Input: part model. Units: mm. Frame: model coordinates. A direction names the side the tool comes from. Round coordinates to 2 decimals unless told otherwise and drop trailing zeros. Order: outer loops, then holes, each group sorted by start corner. A loop starts at its lowest first (then second) coordinate and runs counter-clockwise, first axis right, second up. Notation, with made-up numbers: (35.5, 5.25) -> (86.5, 5.25) arc R8 ccw to (86.5, 14.25) -> close; hole circle Ø2 at (53, 28). An arc over 180 degrees is marked (long way). Use a Markdown table: item, result.
from build123d import *

# Parameters (mm, degrees)
F2_DEPTH = 2.032
F3_DEPTH = 2.54
F5_DEPTH = 25.4
F7_DEPTH = 25.4


with BuildPart() as f2:
    # F0 (on Front) → F2 (new body)
    with BuildSketch(Plane.XZ):
        with BuildLine():
            ThreePointArc((246.888, 191.262), (241.308384, 204.732384), (227.838, 210.312))
            Line((227.838, 210.312), (-227.838, 210.312))
            ThreePointArc((-227.838, 210.312), (-241.308384, 204.732384), (-246.888, 191.262))
            Line((-246.888, 191.262), (-246.888, -191.262))
            ThreePointArc((-246.888, -191.262), (-241.308384, -204.732384), (-227.838, -210.312))
            Line((-227.838, -210.312), (227.838, -210.312))
            ThreePointArc((227.838, -210.312), (241.308384, -204.732384), (246.888, -191.262))
            Line((246.888, -191.262), (246.888, 191.262))
        make_face()
    extrude(amount=F2_DEPTH)

    # F1 (on Front) → F3 (cut)
    with BuildSketch(Plane.XZ):
        with BuildLine():
            Line((223.774, 206.248), (-223.774, 206.248))
            ThreePointArc((-223.774, 206.248), (-237.244384, 200.668384), (-242.824, 187.198))
            Line((-242.824, 187.198), (-242.824, -105.918))
            ThreePointArc((-242.824, -105.918), (-237.244384, -119.388384), (-223.774, -124.968))
            Line((-223.774, -124.968), (223.774, -124.968))
            ThreePointArc((223.774, -124.968), (237.244384, -119.388384), (242.824, -105.918))
            Line((242.824, -105.918), (242.824, 187.198))
            ThreePointArc((242.824, 187.198), (237.244384, 200.668384), (223.774, 206.248))
        make_face()
    extrude(amount=F3_DEPTH, mode=Mode.SUBTRACT)

    # F4 (on Front) → F5 (cut)
    with BuildSketch(Plane.XZ):
        Polygon((-230.124, -134.664931), (-236.474, -134.664931), (-160.274, -200.704931), (-153.924, -200.704931), align=None)
        Polygon((-211.074, -134.664931), (-217.424, -134.664931), (-160.274, -184.194931), (-153.924, -184.194931), align=None)
        Polygon((-230.124, -152.281931), (-236.474, -152.281931), (-180.601308, -200.704931), (-174.251308, -200.704931), align=None)
        Polygon((-230.124, -168.226628), (-236.474, -168.226628), (-198.999035, -200.704931), (-192.649035, -200.704931), align=None)
        Polygon((-230.124, -183.399803), (-236.474, -183.399803), (-216.506545, -200.704931), (-210.156545, -200.704931), align=None)
        Polygon((-160.274, -169.990187), (-153.924, -169.990187), (-194.683911, -134.664931), (-201.033911, -134.664931), align=None)
        Polygon((-160.274, -155.138477), (-153.924, -155.138477), (-177.547322, -134.664931), (-183.897322, -134.664931), align=None)
        Polygon((160.274, -184.194931), (217.424, -134.664931), (211.074, -134.664931), (153.924, -184.194931), align=None)
        Polygon((160.274, -200.704931), (236.474, -134.664931), (230.124, -134.664931), (153.924, -200.704931), align=None)
        Polygon((160.274, -169.990187), (201.033911, -134.664931), (194.683911, -134.664931), (153.924, -169.990187), align=None)
        Polygon((177.547322, -134.664931), (153.924, -155.138477), (160.274, -155.138477), (183.897322, -134.664931), align=None)
        Polygon((198.999035, -200.704931), (236.474, -168.226628), (230.124, -168.226628), (192.649035, -200.704931), align=None)
        Polygon((230.124, -152.281931), (174.251308, -200.704931), (180.601308, -200.704931), (236.474, -152.281931), align=None)
        Polygon((230.124, -183.399803), (210.156545, -200.704931), (216.506545, -200.704931), (236.474, -183.399803), align=None)
    extrude(amount=F5_DEPTH, mode=Mode.SUBTRACT)

    # F6 (on Front) → F7 (cut)
    with BuildSketch(Plane.XZ):
        with BuildLine():
            ThreePointArc((278.867032, 134.112), (282.463983, 140.014539), (283.718, 146.812))
            ThreePointArc((283.718, 146.812), (257.870539, 164.607983), (250.468968, 134.112))
            ThreePointArc((250.468968, 134.112), (264.668, 140.462), (278.867032, 134.112))
        make_face()
        with BuildLine():
            ThreePointArc((278.867032, 134.112), (264.668, 127.762), (250.468968, 134.112))
            ThreePointArc((250.468968, 134.112), (245.618, 121.412), (250.468968, 108.712))
            ThreePointArc((250.468968, 108.712), (264.668, 115.062), (278.867032, 108.712))
            ThreePointArc((278.867032, 108.712), (282.463983, 114.614539), (283.718, 121.412))
            ThreePointArc((283.718, 121.412), (282.463983, 128.209461), (278.867032, 134.112))
        make_face()
        with BuildLine():
            ThreePointArc((278.867032, 108.712), (264.668, 102.362), (250.468968, 108.712))
            ThreePointArc((250.468968, 108.712), (257.870539, 78.216017), (283.718, 96.012))
            ThreePointArc((283.718, 96.012), (282.463983, 102.809461), (278.867032, 108.712))
        make_face()
        with BuildLine():
            ThreePointArc((-250.468968, 134.112), (-246.872017, 140.014539), (-245.618, 146.812))
            ThreePointArc((-245.618, 146.812), (-271.465461, 164.607983), (-278.867032, 134.112))
            ThreePointArc((-278.867032, 134.112), (-264.668, 140.462), (-250.468968, 134.112))
        make_face()
        with BuildLine():
            ThreePointArc((-250.468968, 134.112), (-264.668, 127.762), (-278.867032, 134.112))
            ThreePointArc((-278.867032, 134.112), (-283.718, 121.412), (-278.867032, 108.712))
            ThreePointArc((-278.867032, 108.712), (-264.668, 115.062), (-250.468968, 108.712))
            ThreePointArc((-250.468968, 108.712), (-246.872017, 114.614539), (-245.618, 121.412))
            ThreePointArc((-245.618, 121.412), (-246.872017, 128.209461), (-250.468968, 134.112))
        make_face()
        with BuildLine():
            ThreePointArc((-250.468968, 108.712), (-264.668, 102.362), (-278.867032, 108.712))
            ThreePointArc((-278.867032, 108.712), (-271.465461, 78.216017), (-245.618, 96.012))
            ThreePointArc((-245.618, 96.012), (-246.872017, 102.809461), (-250.468968, 108.712))
        make_face()
    extrude(amount=F7_DEPTH, mode=Mode.SUBTRACT)


solid = f2.part
1) Set-up query: faces 4 (the flat face through (-1, 0, -170)), 5 (the flat face through (-189.25, -1, -159.08)). Return all of +Z, -Z, +X, -X, +Y, -Y with unobstructed straight access to the full face (end or side cutting, diameter ignored); none if empty.
Results found:
| item | result |
|---|---|
| face 4 | +Z, -Z, +X, -X, +Y |
| face 5 | +Y, -Y |
2) Pin query (flat end, axial travel): pin 1 Ø1 at (x, y) = (233, -1.5) entering from -Z; pin 2 Ø0.6 at (x, y) = (-232, -1.5) entering from -Z; pin 3 Ø0.6 at (x, y) = (-234, -1) entering from -Z. Return the tip coordinate at first contact, or that it passes through.
Results found:
| item | result |
|---|---|
| pin 1 | stops at z = -209.73 |
| pin 2 | stops at z = -209.92 |
| pin 3 | stops at z = -209.39 |
3) Cut plane A-A on z = -82.5. Return loops of the section in (x, y).
Results found:
| item | result |
|---|---|
| outline | (-246.89, -2.03) -> (-242.82, -2.03) -> (-242.82, 0) -> (-246.89, 0) -> close; (242.82, -2.03) -> (246.89, -2.03) -> (246.89, 0) -> (242.82, 0) -> close |
4) Pull-direction query (X, two-part tool) for faces 1 (the cylindrical face through (-241.46, -1, -204.58)), 2 (the cylindrical face through (241.46, -1, 204.58)), 3 (the cylindrical face through (237.095, -1.002, -119.536)); classes: +X half, -X half, draft (parallel to the pull), parting line (faces both ways), or undercut.
Results found:
| item | result |
|---|---|
| face 1 | -X half |
| face 2 | +X half |
| face 3 | undercut |
5) Line query: L1, parallel to X at y = -1.3, z = -24; L2, parallel to Z at x = -127.5, y = -0.6; L3, parallel to Z at x = 155, y = -0.6. Output: solid intervals per line, ascending. Write a range as [from, to].
Results found:
| item | result |
|---|---|
| L1 | x = [-246.89, -242.82], [242.82, 246.89] |
| L2 | z = [-210.31, -124.97], [206.25, 210.31] |
| L3 | z = [-210.31, -200.7], [-199.77, -184.19], [-183.26, -169.99], [-169.06, -155.14], [-154.21, -124.97], [206.25, 210.31] |
6) Cut plane B-B on x = 141. Return loops of the section in (y, z).
Results found:
| item | result |
|---|---|
| outline | (-2.03, -210.31) -> (0, -210.31) -> (0, -124.97) -> (-2.03, -124.97) -> close; (-2.03, 206.25) -> (0, 206.25) -> (0, 210.31) -> (-2.03, 210.31) -> close |
7) Cut plane C-C on y = -0.8. Count the separate pieces of the cut face and the enclosed holes in it, and give its area (3 significant figures).
Results found:
| item | result |
|---|---|
| separate pieces | 1 |
| enclosed holes | 15 |
| area | 43,300 mm² |
